Here's how the part is built. I have some questions about the finished solid (model axes, mm). Give positions to 0.01 mm unless a question says otherwise; leave off trailing zeros. Order: outer loops, then holes, each group sorted by start corner. A loop starts at its lowest first (then second) coordinate and runs counter-clockwise, first axis right, second up.
Solid Edge part; units mm, degrees
sketch "Sketch1" plane through (0, 0, 0) normal (0, -1, 0) x (1, 0, 0)
  line L0 (5.8, 35.1) -> (11.8, 35.1)
  arc A0 (11.8, 41.1) -> (11.8, 35.1) centre (11.8, 38.1) cw
  line L1 (11.8, 41.1) -> (5.8, 41.1)
  arc A1 (5.8, 35.1) -> (5.8, 41.1) centre (5.8, 38.1) cw
  line L2 (482.6, 44.45) -> (0, 44.45)
  line L3 (0, 44.45) -> (0, 0)
  line L4 (0, 0) -> (482.6, 0)
  line L5 (482.6, 0) -> (482.6, 44.45)
  arc A2 (5.8, 9.35) -> (5.8, 3.35) centre (5.8, 6.35) ccw
  line L6 (11.8, 3.35) -> (5.8, 3.35)
  arc A3 (11.8, 3.35) -> (11.8, 9.35) centre (11.8, 6.35) ccw
  line L7 (5.8, 9.35) -> (11.8, 9.35)
  circle A4 centre (32.2, 12.7) radius 3
  circle A5 centre (32.2, 31.75) radius 3
  circle A6 centre (105.5, 22.225) radius 3.5
  line L8 (45.3, 8.725) -> (91.3, 8.725)
  line L9 (91.3, 8.725) -> (91.3, 35.725)
  line L10 (91.3, 35.725) -> (45.3, 35.725)
  line L11 (45.3, 35.725) -> (45.3, 8.725)
  line L12 (126.5, 35.725) -> (126.5, 8.725)
  line L13 (126.5, 8.725) -> (172.5, 8.725)
  line L14 (172.5, 8.725) -> (172.5, 35.725)
  line L15 (172.5, 35.725) -> (126.5, 35.725)
  circle A7 centre (186.7, 22.225) radius 3.5
  circle A8 centre (267.9, 22.225) radius 3.5
  line L16 (207.7, 35.725) -> (207.7, 8.725)
  line L17 (207.7, 8.725) -> (253.7, 8.725)
  line L18 (253.7, 8.725) -> (253.7, 35.725)
  line L19 (253.7, 35.725) -> (207.7, 35.725)
  line L20 (288.9, 35.725) -> (288.9, 8.725)
  line L21 (288.9, 8.725) -> (334.9, 8.725)
  line L22 (334.9, 8.725) -> (334.9, 35.725)
  line L23 (334.9, 35.725) -> (288.9, 35.725)
  circle A9 centre (349.1, 22.225) radius 3.5
  line L24 (370.1, 35.725) -> (370.1, 8.725)
  line L25 (370.1, 8.725) -> (416.1, 8.725)
  line L26 (416.1, 8.725) -> (416.1, 35.725)
  line L27 (416.1, 35.725) -> (370.1, 35.725)
  circle A10 centre (430.3, 22.225) radius 3.5
  arc A11 (476.8, 35.1) -> (476.8, 41.1) centre (476.8, 38.1) ccw
  line L28 (470.8, 41.1) -> (476.8, 41.1)
  arc A12 (470.8, 41.1) -> (470.8, 35.1) centre (470.8, 38.1) ccw
  line L29 (476.8, 35.1) -> (470.8, 35.1)
  circle A13 centre (450.4, 31.75) radius 3
  line L30 (470.8, 3.35) -> (476.8, 3.35)
  arc A14 (476.8, 9.35) -> (476.8, 3.35) centre (476.8, 6.35) cw
  line L31 (476.8, 9.35) -> (470.8, 9.35)
  arc A15 (470.8, 3.35) -> (470.8, 9.35) centre (470.8, 6.35) cw
  circle A16 centre (450.4, 12.7) radius 3
extrude "Protrusion1" add sketch "Sketch1" along normal blind 3
Q1. If we section it at B-B on y = -2.35: Give the number of separate pieces and of enclosed holes in the cut face, plus the area to 3 significant figures.
Filled sheet:
separate pieces: 1
enclosed holes: 18
area: 14,700 mm2
Q2. I'm going to push a flat-ended pin straight in: P1, Ø8, axis at x = 450.4, z = 12.7, coming from the -Y side. Where does the tip first touch, or does it pass through?
Filled sheet:
P1: stops at y = -3
Q3. If we section it at A-A on x = 76: List the corners of the cut face in (y, z) for me (3 decimals).
Filled sheet:
outline: (-3, 0) - (0, 0) - (0, 8.725) - (-3, 8.725) - close; (-3, 35.725) - (0, 35.725) - (0, 44.45) - (-3, 44.45) - close
Q4. I need wall thicknesses on L1, parallel to X at y = -0.9, z = 35; L2, parallel to Z at x = 32.2, y = -0.9; L3, parallel to Z at x = 349.1, y = -1.5 (3 decimals). Which ranges of each line are inside material? Lowest first, please.
Filled sheet:
L1: x = 0 to 45.3, 91.3 to 126.5, 172.5 to 207.7, 253.7 to 288.9, 334.9 to 370.1, 416.1 to 482.6
L2: z = 0 to 9.7, 15.7 to 28.75, 34.75 to 44.45
L3: z = 0 to 18.725, 25.725 to 44.45
